Geometry: final body of the model. Coordinates: model frame, mm. A direction names the side the tool comes from. Give positions to 0.01 mm unless a question says otherwise; leave off trailing zeros. Loops run counter-clockwise (first coordinate to the right, second up) from the corner with the lowest first, then second, coordinate; pieces in that order, holes last. Notation, with made-up numbers: (45.5, 74) -> (72.5, 74) arc R35 cw to (72.5, 107) -> close; hole circle Ø5 at (-5, 85.25). An arc over 180 degrees is marked (long way). Answer in a Markdown table with one row per item. Add a question column.
1) Access query for faces 4 (the cylindrical face through (-1.301, -57.857, 3.042)), 5 (the cylindrical face through (16.953, 24.501, 2.958)). Directions: +Z, -Z, +X, -X, +Y, -Y. A direction counts if a zero-diameter tool reaches every point of the face in a straight line with its end or side. Return the directions, or none.
2) Line query: line 1 (Y direction, x = 1, z = 1.2); line 2 (Y direction, x = 0, z = 2); line 3 (X direction, y = -53, z = 4.15). Output: solid intervals per line, ascending. Write a range as from..to.
3) Section query C-C (y = 52). Return the cut outline in (x, z).
4) Section query B-B (z = 1.25). Return the cut outline in (x, y).
5) Draft query along Y for faces 1 (the cylindrical face through (35.062, -36.483, 2.958)), 2 (the flat face through (30, -1, 0)), 3 (the cylindrical face through (0, 55, 3)). Return one class per face: +Y half, -Y half, draft (parallel to the pull), parting line (faces both ways), or undercut.
6) First-contact query: P1, Ø7, axis at x = 0, y = 52, coming from the +Z side; P2, Ø2, axis at x = 26, z = 5, coming from the +Y side; P3, Ø1.5, axis at x = 23, z = 5, coming from the +Y side; P4, Ø1.5, axis at y = -12, z = 4, coming from the -X side. Flat tips, straight axial feed; report the tip coordinate or a pass-through.
7) Section query D-D (x = 16). Return the cut outline in (y, z), plus the area to 3 significant figures.
8) Section query A-A (x = 0). Return the cut outline in (y, z).
```python
from build123d import *

# Parameters (mm, degrees)
EXTRUDE_1_DEPTH     = 6
SKETCH_2_R          = 9
EXTRUDE_2_DEPTH     = 6
SKETCH_3_R          = 6
SKETCH_3_R_2        = 3
CUT_EXTRUDE_1_DEPTH = 6


with BuildPart() as part:
    # 草图1 → 凸台-拉伸1 (new body)
    with BuildSketch(Plane.XY):
        with BuildLine():
            ThreePointArc((0.601101389, -57.969813826), (33.334648413, -39.063402424), (40.851101389, -2.016939333))
            ThreePointArc((40.851101389, -2.016939333), (27.330534013, 30.544098151), (3.708244246, 56.716876574))
            ThreePointArc((3.708244246, 56.716876574), (-4.716876574, 55.708244246), (-3.708244246, 47.283123426))
            ThreePointArc((-3.708244246, 47.283123426), (17.188396702, 24.130280975), (29.148898611, -4.673713722))
            ThreePointArc((29.148898611, -4.673713722), (23.593259455, -32.055882093), (-0.601101389, -46.030186174))
            ThreePointArc((-0.601101389, -46.030186174), (-5.969813826, -52.601101389), (0.601101389, -57.969813826))
        make_face()
    extrude(amount=EXTRUDE_1_DEPTH)

    # 草图2 → 凸台-拉伸2 (add)
    with BuildSketch(Plane.XY.offset(6)):
        with Locations((0, -52)):
            Circle(SKETCH_2_R)
    extrude(amount=-EXTRUDE_2_DEPTH)

    # 草图3 → 切除-拉伸1 (cut)
    with BuildSketch(Plane.XY.offset(6)):
        with Locations((0, -52)):
            Circle(SKETCH_3_R)
        with Locations((0, 52)):
            Circle(SKETCH_3_R_2)
    extrude(amount=-CUT_EXTRUDE_1_DEPTH, mode=Mode.SUBTRACT)


solid = part.part
```
Evaluation:
| question | item | result |
|---|---|---|
| 1 | face 4 | +Z, -Z |
| 1 | face 5 | +Z, -Z, -X |
| 2 | line 1 | -60.94..-57.92, -46.08..-43.06, 43.32..49.17, 54.83..57.92 |
| 2 | line 2 | -61..-58, -46..-43, 44.21..49, 55..58 |
| 2 | line 3 | -8.94..-5.92, 5.92..17.24 |
| 3 | outline | (-6, 0) -> (-3, 0) -> (-3, 6) -> (-6, 6) -> close; (3, 0) -> (9.29, 0) -> (9.29, 6) -> (3, 6) -> close |
| 4 | outline | (-3.71, 47.28) arc R92 cw to (29.15, -4.67) arc R34 cw to (5.47, -44.85) arc R9 ccw (long way) to (7.68, -56.69) arc R46 ccw to (40.85, -2.02) arc R104 ccw to (3.71, 56.72) arc R6 ccw to start; hole circle Ø12 at (0, -52); hole circle Ø6 at (0, 52) |
| 5 | face 1 | parting line |
| 5 | face 2 | draft |
| 5 | face 3 | undercut |
| 6 | P1 | z = 6 |
| 6 | P2 | y = 34.07 |
| 6 | P3 | y = 37.86 |
| 6 | P4 | x = 29.98 |
| 7 | outline | (-53.62, 0) -> (-39.69, 0) -> (-39.69, 6) -> (-53.62, 6) -> close; (25.96, 0) -> (45.34, 0) -> (45.34, 6) -> (25.96, 6) -> close |
| 7 | area | 200 mm² |
| 8 | outline | (-61, 0) -> (-58, 0) -> (-58, 6) -> (-61, 6) -> close; (-46, 0) -> (-43, 0) -> (-43, 6) -> (-46, 6) -> close; (44.21, 0) -> (49, 0) -> (49, 6) -> (44.21, 6) -> close; (55, 0) -> (58, 0) -> (58, 6) -> (55, 6) -> close |
